The listing builds one solid part. Answer for the finished solid, in the listing's coordinates (mm). Round coordinates to 2 decimals unless told otherwise and drop trailing zeros. Loops run counter-clockwise (first coordinate to the right, second up) from the corner with the lowest first, then second, coordinate; pieces in that order, holes last. Notation, with made-up numbers: M 16,62.25 L 33,62.25 A28 ccw 33,90.25 Z; hole C -15,-33.5 d1. An arc over 180 degrees is marked long. Answer as a JSON object with one key per item and string values.
Autodesk Inventor part; units mm, degrees
ref_plane "YZ Plane" through (0, 0, 0) normal (1, 0, 0) x (0, 1, 0)
ref_plane "XZ Plane" through (0, 0, 0) normal (0, 1, 0) x (-1, 0, 0)
ref_plane "XY Plane" through (0, 0, 0) normal (0, 0, 1) x (1, 0, 0)
sketch "Sketch1" plane through (0, 0, 0) normal (0, 1, 0) x (-1, 0, 0)
  line L0 (6, 6) -> (-6, 6)
  line L1 (-6, 6) -> (-6, -6)
  line L2 (-6, -6) -> (6, -6)
  line L3 (6, -6) -> (6, 6)
  line L4 (6, 6) -> (-6, -6) construction
  line L5 (-6, 6) -> (6, -6) construction
  point P0 (0, 0)
  dimension "d0" = 12
  dimension "d1" = 12
extrude "Extrusion1" add sketch "Sketch1" along normal blind 2
sketch "Sketch2" plane through (0, 2, 0) normal (0, 1, 0) x (1, 0, 0)
  line L0 (-0.0927, -0.2032) -> (0.0511, -0.2032)
  line L1 (0.0511, -0.2032) -> (-0.1769, -0.0781)
  line L2 (-0.1769, -0.0781) -> (-0.1593, -0.3245)
  line L3 (-0.1593, -0.3245) -> (-0.0927, -0.2032)
  line L4 (-0.0811, 0.2563) -> (-0.126, 0.1039)
  line L5 (-0.126, 0.1039) -> (-0.0159, 0.0999)
  line L6 (-0.0159, 0.0999) -> (-0.0811, 0.2563)
  line L7 (0.315, -0.1506) -> (0.1499, 0.28)
  line L8 (0.1499, 0.28) -> (0.0261, 0.2325)
  line L9 (0.0261, 0.2325) -> (0.1912, -0.198)
  line L10 (0.1912, -0.198) -> (0.315, -0.1506)
  line L11 (0.315, -0.1506) -> (0.0261, 0.2325) construction
  line L12 (0.1499, 0.28) -> (0.1912, -0.198) construction
  point P0 (0, 0)
  point P1 (0.1705, 0.041)
extrude "Extrusion2" cut sketch "Sketch2" along normal mid plane 0.06 contours L3 L2 L1 L0
extrude "Extrusion3" add sketch "Sketch2" along normal blind 0.03 contours L6 L5 L4
extrude "Extrusion4" add sketch "Sketch2" along normal blind 0.02 contours L10 L9 L8 L7
draft "FaceDraft1" angle 20 pull direction (-0.9337322, 0, 0.3579724) faces at (0.2187, 2.02, 0.0229) fixed edges at (0.1086, 2.02, -0.0173)
properties part number "example_sample"
Item 1: The part is cut by section A-A (z = 1). Give the vertices of the cut face in (x, y).
Values follow:
{"outline": "M -6,0 L 6,0 L 6,2 L -6,2 Z"}
Item 2: The part is cut by section B-B (x = -5). Give the vertices of the cut face in (y, z), then the cut area to 3 significant figures.
Values follow:
{"outline": "M 0,-6 L 2,-6 L 2,6 L 0,6 Z", "area": "24.0 mm^2"}
Item 3: A flat-ended cylindrical pin translates along its axis: P1, Ø1, axis at x = 2, z = 3.5, coming from the +Y side. Find the tip coordinate at first contact, or state that the pin passes through.
Values follow:
{"P1": "y = 2"}
Item 4: A straight line is drawn through the part: line 1 (Y direction, x = 5.25, z = -2.75). Find the intervals that lie inside material, in ascending order.
Values follow:
{"line 1": "0 to 2"}
